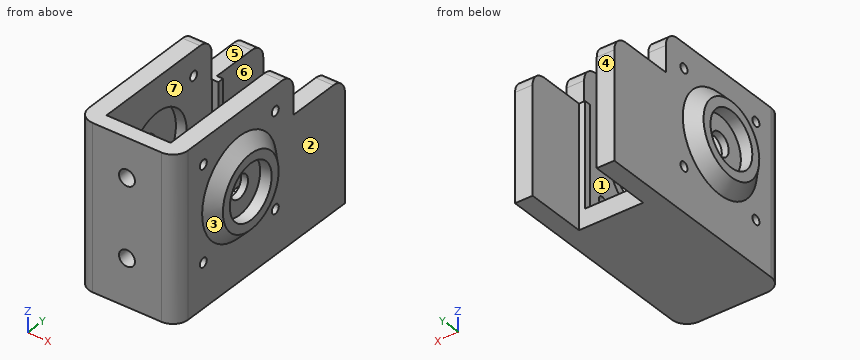
```python
from build123d import *

# Parameters (mm, degrees)
F1_DEPTH       = 16.25
F2_R           = 3.75
F3_DEPTH       = 16.251
F3_DEPTH_BACK  = 16.251
F4_W           = 21
F4_H           = 67.5
F5_DEPTH       = 47.5
F10_W          = 21
F10_H          = 6
F11_DEPTH      = 20
F12_W          = 2
F12_H          = 2
F13_DEPTH      = 34
F14_R          = 12.5
F15_DEPTH      = 14
F16_R          = 5
F17_R          = 1.5
F18_DEPTH      = 20.001
F18_DEPTH_BACK = 20.001
F19_R          = 2.6162
F20_DEPTH      = 25


with BuildPart() as f1:
    # F0 (on Right) → F1 (new body, symmetric)
    with BuildSketch(Plane.YZ):
        with BuildLine():
            Line((0, 53.5), (0, 0))
            Line((0, 0), (72.5, 0))
            Line((72.5, 0), (72.5, 35))
            ThreePointArc((72.5, 35), (71.0355339059, 38.5355339059), (67.5, 40))
            Line((67.5, 40), (50.3, 40))
            Line((50.3, 40), (50.3, 48.5))
            ThreePointArc((50.3, 48.5), (48.8355339059, 52.0355339059), (45.3, 53.5))
            Line((45.3, 53.5), (0, 53.5))
        make_face()
    extrude(amount=F1_DEPTH, both=True)

    # F2 (on Right) → F3 (cut, two sides)
    with BuildSketch(Plane.YZ) as f3_sk:
        with Locations((27, 30)):
            Circle(F2_R)
    extrude(amount=-F3_DEPTH, mode=Mode.SUBTRACT)
    extrude(f3_sk.sketch, amount=F3_DEPTH_BACK, mode=Mode.SUBTRACT)

    # F4 (on face) → F5 (cut)
    with BuildSketch(Plane.XY.offset(53.5)):
        with Locations((0, 38.75)):
            Rectangle(F4_W, F4_H)
    extrude(amount=-F5_DEPTH, mode=Mode.SUBTRACT)

    # F7 (on offset) → F8 (revolve)
    with BuildSketch(Plane.XZ.offset(-27)):
        Polygon((20, 42), (16.25, 46), (16.25, 39), (20, 39), align=None)
    revolve(axis=Axis((16.25, 27, 30), (1, 0, 0)))

    # F9: F1 across plane


with BuildPart() as f1_1:
    add(f1.part)
    add(f1.part.mirror(Plane.YZ))

    # F10 (on face) → F11 (cut)
    with BuildSketch(Plane(origin=(0, 72.5, 0), x_dir=(-1, 0, 0), z_dir=(0, 1, 0))):
        with Locations((0, 3)):
            Rectangle(F10_W, F10_H)
    extrude(amount=-F11_DEPTH, mode=Mode.SUBTRACT)

    # F12 (on face) → F13 (join, through all)
    with BuildSketch(Plane.XY.offset(6)):
        with Locations((-9.5, 51.5)):
            Rectangle(F12_W, F12_H)
        with Locations((9.5, 51.5)):
            Rectangle(F12_W, F12_H)
    extrude(amount=F13_DEPTH)

    # F14 (on Right) → F15 (cut, symmetric)
    with BuildSketch(Plane.YZ):
        with Locations((27, 30)):
            Circle(F14_R)
    extrude(amount=F15_DEPTH, both=True, mode=Mode.SUBTRACT)

    # F16
    f16_edges = [f1_1.edges().sort_by_distance(p)[0] for p in [
        (16.25, 0, 26.75),
        (-16.25, 0, 26.75),
    ]]
    fillet(f16_edges, radius=F16_R)

    # F17 (on Right) → F18 (cut, two sides)
    with BuildSketch(Plane.YZ) as f18_sk:
        with Locations((11.5, 45.5)):
            Circle(F17_R)
        with Locations((11.5, 14.5)):
            Circle(F17_R)
        with Locations((42.5, 14.5)):
            Circle(F17_R)
        with Locations((42.5, 45.5)):
            Circle(F17_R)
    extrude(amount=-F18_DEPTH, mode=Mode.SUBTRACT)
    extrude(f18_sk.sketch, amount=F18_DEPTH_BACK, mode=Mode.SUBTRACT)

    # F19 (on face) → F20 (cut)
    with BuildSketch(Plane.XZ):
        with Locations((0, 40.8)):
            Circle(F19_R)
        with Locations((0, 15.4)):
            Circle(F19_R)
    extrude(amount=-F20_DEPTH, mode=Mode.SUBTRACT)


solid = f1_1.part
```
Input: part model. Units: mm. Frame: model coordinates. Face numbers are marked on the shaded views. A direction names the side the tool comes from. Round coordinates to 2 decimals unless told otherwise and drop trailing zeros. Loops run counter-clockwise (first coordinate to the right, second up) from the corner with the lowest first, then second, coordinate; pieces in that order, holes last. Notation, with made-up numbers: (3.5, -18.5) -> (18.5, -18.5) arc R25 ccw to (18.5, 14.5) -> close; hole circle Ø3 at (69.25, -22). An arc over 180 degrees is marked (long way). One line per item, written item: value.
(1) Section D-D (x = 12.5). Return the cut outline in (y, z), plus the area to 3 significant figures.
Geometry check:
outline: (0.16, 0) -> (72.5, 0) -> (72.5, 35) arc R5 ccw to (67.5, 40) -> (50.3, 40) -> (50.3, 48.5) arc R5 ccw to (45.3, 53.5) -> (0.16, 53.5) -> close; hole circle Ø3 at (11.5, 14.5); hole circle Ø3 at (11.5, 45.5); hole circle Ø25 at (27, 30); hole circle Ø3 at (42.5, 14.5); hole circle Ø3 at (42.5, 45.5)
area: 3,040 mm2
(2) Mould query, pull axis Y, two halves, no side actions, for the marked faces 1, 2, 3 and 4. Classes: pulls with the +Y half, pulls with the -Y half, needs draft (parallel to the pull), parting line crosses it, or undercut.
Geometry check:
face 1: undercut
face 2: needs draft
face 3: parting line crosses it
face 4: pulls with the +Y half
(3) Section C-C (y = 27). Give the number of separate pieces and of enclosed holes in the cut face, plus the area to 4 significant figures.
Geometry check:
separate pieces: 3
enclosed holes: 0
area: 607.5 mm2
(4) Section B-B (z = 7). Return the cut outline in (x, y).
Geometry check:
outline: (-16.25, 5) arc R5 ccw to (-11.25, 0) -> (11.25, 0) arc R5 ccw to (16.25, 5) -> (16.25, 72.5) -> (10.5, 72.5) -> (10.5, 52.5) -> (8.5, 52.5) -> (8.5, 50.5) -> (10.5, 50.5) -> (10.5, 5) -> (-10.5, 5) -> (-10.5, 50.5) -> (-8.5, 50.5) -> (-8.5, 52.5) -> (-10.5, 52.5) -> (-10.5, 72.5) -> (-16.25, 72.5) -> close
(5) Material intervals for line 1 (Z direction, x = -12.25, y = 42.5); line 2 (Z direction, x = 0, y = 3.3); line 3 (X direction, y = 58.5, z = 14), sorted ascending. Write a range as [from, to].
Geometry check:
line 1: [0, 13], [16, 44], [47, 53.5]
line 2: [0, 12.78], [18.02, 38.18], [43.42, 53.5]
line 3: [-16.25, -10.5], [10.5, 16.25]
(6) Section A-A (x = 0). Return the cut outline in (y, z).
Geometry check:
outline: (0, 0) -> (52.5, 0) -> (52.5, 6) -> (5, 6) -> (5, 12.78) -> (0, 12.78) -> close; (0, 18.02) -> (5, 18.02) -> (5, 38.18) -> (0, 38.18) -> close; (0, 43.42) -> (5, 43.42) -> (5, 53.5) -> (0, 53.5) -> close
(7) Set-up query: the marked faces 5, 6 and 7. Return all of +Z, -Z, +X, -X, +Y, -Y with unobstructed straight access to the full face (end or side cutting, diameter ignored); none if empty.
Geometry check:
face 5: +Z, +X, -X, +Y
face 6: +Z, -Z, +Y
face 7: +Z
(8) Pin query (flat end, axial travel): pin 1 (5 mm diameter, centred on x = 8.5, z = 39.5, fed in from +Y); pin 2 (6.5 mm diameter, centred on x = -4, z = 31, fed in from +Y); pin 3 (2.5 mm diameter, centred on x = -11, y = 62, fed in from +Z); pin 4 (23 mm diameter, centred on y = 34, z = 26, fed in from +X). Return the tip coordinate at first contact, or that it passes through.
Geometry check:
pin 1: y = 71.5
pin 2: y = 5
pin 3: z = 40
pin 4: x = 20
